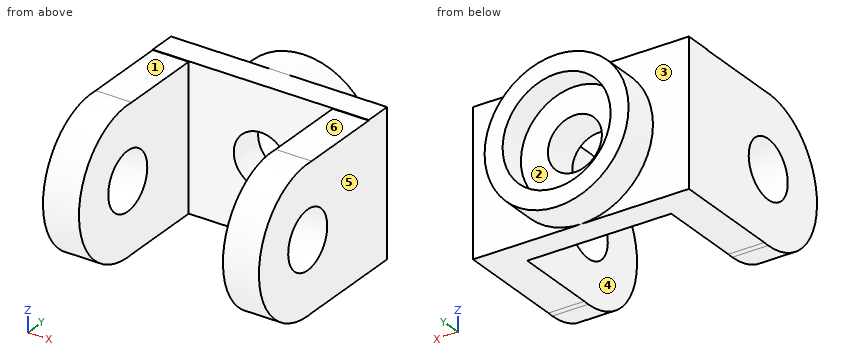
from build123d import *

# Parameters (mm, degrees)
SKETCH1_W           = 120
SKETCH1_H           = 80
BOSS_EXTRUDE1_DEPTH = 15
SKETCH2_R           = 40
BOSS_EXTRUDE2_DEPTH = 20
SKETCH3_R           = 30
CUT_EXTRUDE1_DEPTH  = 15
SKETCH4_R           = 15
CUT_EXTRUDE2_DEPTH  = 75.833147735
BOSS_EXTRUDE3_DEPTH = 20
SKETCH6_R           = 16
CUT_EXTRUDE3_DEPTH  = 156.274782914


with BuildPart() as part:
    # Sketch1 → Boss-Extrude1 (new body)
    with BuildSketch(Plane(origin=(0, 0, 0), x_dir=(1, 0, 0), z_dir=(0, 1, 0))):
        Rectangle(SKETCH1_W, SKETCH1_H)
    extrude(amount=BOSS_EXTRUDE1_DEPTH)

    # Sketch2 → Boss-Extrude2 (add)
    with BuildSketch(Plane(origin=(0, 15, 0), x_dir=(1, 0, 0), z_dir=(0, 1, 0))):
        with Locations(Location((0, 0, 0), (0, 0, 270))):
            Circle(SKETCH2_R)
    extrude(amount=BOSS_EXTRUDE2_DEPTH)

    # Sketch3 → Cut-Extrude1 (cut)
    with BuildSketch(Plane(origin=(0, 35, 0), x_dir=(1, 0, 0), z_dir=(0, 1, 0))):
        with Locations(Location((0, 0, 0), (0, 0, 270))):
            Circle(SKETCH3_R)
    extrude(amount=-CUT_EXTRUDE1_DEPTH, mode=Mode.SUBTRACT)

    # Sketch4 → Cut-Extrude2 (cut, through all)
    with BuildSketch(Plane(origin=(0, 20, 0), x_dir=(1, 0, 0), z_dir=(0, 1, 0))):
        with Locations(Location((0, 0, 0), (0, 0, 270))):
            Circle(SKETCH4_R)
    extrude(amount=-CUT_EXTRUDE2_DEPTH, mode=Mode.SUBTRACT)

    # Sketch5 → Boss-Extrude3 (add)
    with BuildSketch(Plane(origin=(60, 0, 0), x_dir=(0, 0, -1), z_dir=(1, 0, 0))):
        with BuildLine():
            Line((40, -46.802277462), (40, 0))
            Line((40, 0), (-39.743954519, 0))
            Line((-39.743954519, 0), (-39.743954519, -46.802277462))
            ThreePointArc((-39.743954519, -46.802277462), (0.128022741, -10), (40, -46.802277462))
        make_face()
        with BuildLine():
            ThreePointArc((40.128022741, -50), (40.096004241, -48.399857877), (40, -46.802277462))
            Line((40, -46.802277462), (40, -50))
            Line((40, -50), (-39.743954519, -50))
            Line((-39.743954519, -50), (-39.743954519, -46.802277462))
            ThreePointArc((-39.743954519, -46.802277462), (-1.472119382, -89.9679815), (40.128022741, -50))
        make_face()
        with BuildLine():
            Line((40, -50), (40, -46.802277462))
            ThreePointArc((40, -46.802277462), (0.128022741, -10), (-39.743954519, -46.802277462))
            Line((-39.743954519, -46.802277462), (-39.743954519, -50))
            Line((-39.743954519, -50), (40, -50))
        make_face()
    boss_extrude3 = extrude(amount=-BOSS_EXTRUDE3_DEPTH)

    # Sketch6 → Cut-Extrude3 (cut, through all)
    with BuildSketch(Plane(origin=(60, 0, 0), x_dir=(0, 0, -1), z_dir=(1, 0, 0))):
        with Locations((0.128022741, -50)):
            Circle(SKETCH6_R)
    cut_extrude3 = extrude(amount=-CUT_EXTRUDE3_DEPTH, mode=Mode.SUBTRACT)

    # Mirror2: Boss-Extrude3, Cut-Extrude3 across plane
    add(boss_extrude3.mirror(Plane(origin=(0, 0, 0), x_dir=(0, 0, 1), z_dir=(1, 0, 0))))
    add(cut_extrude3.mirror(Plane(origin=(0, 0, 0), x_dir=(0, 0, 1), z_dir=(1, 0, 0))), mode=Mode.SUBTRACT)


solid = part.part
Verification items for the finished model (mm, model axes). Face numbers are marked on the shaded views. A direction names the side the tool comes from. Give positions to 0.01 mm unless a question says otherwise; leave off trailing zeros. Loops run counter-clockwise (first coordinate to the right, second up) from the corner with the lowest first, then second, coordinate; pieces in that order, holes last.
1) Depth check by flat-ended pin: pin 1 Ø8 at (x, z) = (-2, -22.5) entering from +Y; pin 2 Ø6 at (x, y) = (-53, -22) entering from +Z; pin 3 Ø12 at (x, z) = (5.5, -9.5) entering from -Y. Enter the tip coordinate at first touch or a pass-through.
2) Draft check along X on the marked faces 4, 5 and 6. Enter one of: pulls with the +X half, pulls with the -X half, needs draft (parallel to the pull), parting line crosses it, or undercut.
3) Set-up check for the marked faces 1, 2 and 3: record each of +Z, -Z, +X, -X, +Y, -Y from which the full face is reachable in a straight line by a thin tool's end or side.
4) Sectioned sample at B-B, the plane z = 7. Enter the section's corners in (x, y).
5) Sectioned sample at C-C, the plane x = -45. Enter the section's corners in (y, z).
6) Sectioned sample at D-D, the plane x = -11.5. Enter the section's corners in (y, z).
7) Thickness scan on line 1 along X through (y, z) = (-50, 30.5); line 2 along X through (y, z) = (13.25, 0); line 3 along Y through (x, z) = (23, 12). Record the ranges inside material, lowest first.
8) Sectioned sample at A-A, the plane y = -19. Enter the section's corners in (x, z), then the cut area to 3 significant figures.
Answers:
1. pin 1: stops at y = 20
1. pin 2: stops at z = 39.74
1. pin 3: stops at y = 0
2. face 4: undercut
2. face 5: pulls with the +X half
2. face 6: needs draft
3. face 1: +Z, +X, -X
3. face 2: +Y
3. face 3: -X, +Y
4. outline: (-60, -89.36) - (-40, -89.36) - (-40, -64.32) - (-60, -64.32) - close; (-60, -35.68) - (-40, -35.68) - (-40, 0) - (-13.27, 0) - (-13.27, 20) - (-29.17, 20) - (-29.17, 35) - (-39.38, 35) - (-39.38, 15) - (-60, 15) - close; (13.27, 0) - (40, 0) - (40, -35.68) - (60, -35.68) - (60, 15) - (39.38, 15) - (39.38, 35) - (29.17, 35) - (29.17, 20) - (13.27, 20) - close; (40, -89.36) - (60, -89.36) - (60, -64.32) - (40, -64.32) - close
5. outline: (-46.8, -40) - (15, -40) - (15, 40) - (0, 40) - (0, 39.74) - (-46.8, 39.74) arc R40 ccw (long way) to start; hole circle Ø32 at (-50, -0.13)
6. outline: (0, -40) - (15, -40) - (15, -38.31) - (35, -38.31) - (35, -27.71) - (20, -27.71) - (20, -9.63) - (0, -9.63) - close; (0, 9.63) - (20, 9.63) - (20, 27.71) - (35, 27.71) - (35, 38.31) - (15, 38.31) - (15, 40) - (0, 40) - close
7. line 1: x = -60 to -40, 40 to 60
7. line 2: x = -60 to -15, 15 to 60
7. line 3: y = 0 to 20
8. outline: (-60, -40) - (-40, -40) - (-40, 39.74) - (-60, 39.74) - close; (40, -40) - (60, -40) - (60, 39.74) - (40, 39.74) - close
8. area: 3,190 mm2
